```python
from build123d import *

# Parameters (mm, degrees)
SKETCH_2_R          = 2.5
SKETCH_2_W          = 13.733275584
SKETCH_2_H          = 7.68132945
CUT_EXTRUDE_1_DEPTH = 15


with BuildPart() as part:
    # Эскиз1 → Повернуть1 (revolve)
    with BuildSketch(Plane.XY, mode=Mode.PRIVATE) as revolve_1_sk:
        Polygon((0, 0), (-1.057961884, 6), (-10.057961884, 6), (-10.057961884, 10), (-20.057961884, 10), (-20.057961884, 0), align=None)
    revolve(revolve_1_sk.sketch.rotate(Axis((0, 0, 0), (-1, 0, 0)), 90), axis=Axis((0, 0, 0), (-1, 0, 0)))

    # Эскиз2 → Вырез-Вытянуть1 (cut, symmetric)
    with BuildSketch(Plane.XY):
        with Locations((-15.057961884, 0)):
            Circle(SKETCH_2_R)
        with Locations((-14.936439869, -11.840664725)):
            Rectangle(SKETCH_2_W, SKETCH_2_H)
        with Locations((-14.936439869, 11.840664725)):
            Rectangle(SKETCH_2_W, SKETCH_2_H)
    extrude(amount=CUT_EXTRUDE_1_DEPTH, both=True, mode=Mode.SUBTRACT)


solid = part.part
```
CAD build for the part. Positions are in the model's coordinates, mm. A direction names the side the tool comes from. Coordinates: 2 decimals unless noted, no trailing zeros. Order: outer loops, then holes, each group sorted by start corner. A loop starts at its lowest first (then second) coordinate and runs counter-clockwise, first axis right, second up. Notation, with made-up numbers: M 6.5,-19.75 L 53.5,-19.75 A17 ccw 53.5,6.25 Z; hole C -27,13 d10. An arc over 180 degrees is marked long. Answer as CSV lines item,"result".
1) Cut at B-B (x = -5.25). List the corners of the cut face in (y, z), then the cut area to 3 significant figures.
Verdict:
outline,"C 0,0 d12"
area,"113 mm2"
2) Cut at A-A (z = 6.75). List the corners of the cut face in (x, y), then the cut area to 3 significant figures.
Verdict:
outline,"M -20.06,-7.38 L -10.06,-7.38 L -10.06,7.38 L -20.06,7.38 Z; hole C -15.06,0 d5"
area,"128 mm2"
3) Cut at C-C (x = -12.25). List the corners of the cut face in (y, z).
Verdict:
outline,"M -8,-6 A10 ccw 8,-6 L 8,6 A10 ccw -8,6 Z"
4) Mould opens along X. For faces 3 (the flat face through (-20.058, 0, 0)), 4 (the cylindrical face through (-17.042, -1.521, 0.139)), 5 (the flat face through (-10.058, 0, 7)) say: released by +X, released by -X, zero draft, split by the parting line, or undercut.
Verdict:
face 3,"released by -X"
face 4,"undercut"
face 5,"released by +X"
5) Flat gauge pins, fed straight in: P1, Ø8, axis at y = -2, z = -4, coming from the +X side; P2, Ø1.5, axis at x = -5.5, y = -0.5, coming from the -Z side; P3, Ø2, axis at x = -4, y = -2.5, coming from the +Z side; P4, Ø5, axis at x = -10.5, y = 1.5, coming from the +Z side. Where does each tip first touch, or does it go through?
Verdict:
P1,"x = -0.08"
P2,"z = -6"
P3,"z = 5.81"
P4,"z = 10"
6) Drill centre lines: L1, parallel to X at y = -7.5, z = -1; L2, parallel to X at y = 1, z = 0; L3, parallel to X at y = 0, z = 3. Where is each one in solid material? Low to high. Write a range as from..to.
Verdict:
L1,"-20.06..-10.06"
L2,"-20.06..-17.35, -12.77..-0.18"
L3,"-20.06..-17.56, -12.56..-0.53"
7) 3-axis set-ups, long thin cutter, end or side, ignore diameter. For faces 1 (the cylindrical face through (-5.621, -1.802, -5.723)), 2 (the flat face through (-15, -8, 0)): which of +Z, -Z, +X, -X, +Y, -Y reach the whole face in a straight line?
Verdict:
face 1,"+X"
face 2,"+Z, -Z, +X, -X, -Y"
